Build history of the part. All positions in model axes, mm. Face numbers are marked on the shaded views. Round coordinates to 2 decimals unless told otherwise and drop trailing zeros. Loops run counter-clockwise (first coordinate to the right, second up) from the corner with the lowest first, then second, coordinate; pieces in that order, holes last. Notation, with made-up numbers: (20.25, 81.25) - (50.25, 81.25) arc R24 cw to (50.25, 91.25) - close; hole circle Ø5 at (43, 89.5). An arc over 180 degrees is marked (long way). Use one line per item in the form item = value. Start each with the question number.
Q1. Saw through at A-A (z = 0). Give the cut face in (x, y).
Q2. Saw through at B-B (x = 0). Give the cut face in (y, z).
Q3. Drill centre lines: line 1 (Y direction, x = -22, z = -29.5); line 2 (Z direction, x = 10.5, y = 2.75); line 3 (X direction, y = 2.5, z = 14). Where is each one in solid material? Low to high.
Q4. Mould opens along X. For the marked faces 1, 2 and 3 say: released by +X, released by -X, zero draft, split by the parting line, or undercut.
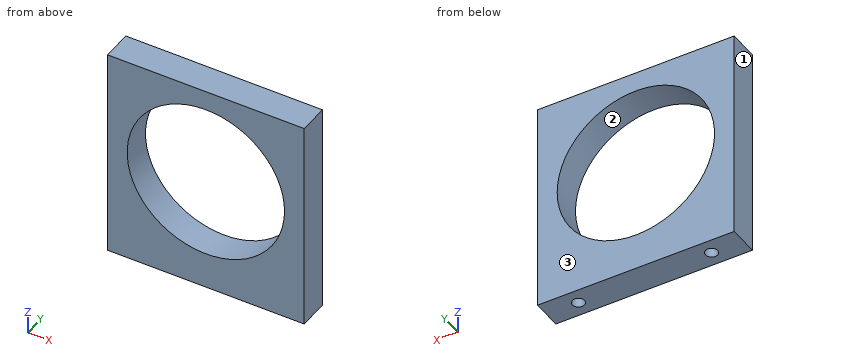
```python
from build123d import *

# Parameters (mm, degrees)
F0_W     = 65
F0_H     = 70.5
F0_R     = 26
F1_DEPTH = 5
F3_D     = 4
F3_DEPTH = 15
F3_TIP   = 1.2017212381


with BuildPart() as f1:
    # F0 (on Front) → F1 (new body, symmetric)
    with BuildSketch(Plane.XZ):
        with Locations((0, -2.75)):
            Rectangle(F0_W, F0_H)
        Circle(F0_R, mode=Mode.SUBTRACT)
    extrude(amount=F1_DEPTH, both=True)

    # F3
    with Locations(Plane(origin=(0, 0, -38), x_dir=(1, 0, 0), z_dir=(0, 0, -1))):
        with Locations((-22, 0), (22, 0)):
            Hole(F3_D / 2, depth=F3_DEPTH)
            with Locations((0, 0, -(F3_DEPTH + F3_TIP / 2))):  # 118° drill point
                Cone(0, F3_D / 2, F3_TIP, mode=Mode.SUBTRACT)


solid = f1.part
```
Report:
q1.outline = (-32.5, -5) - (-26, -5) - (-26, 5) - (-32.5, 5) - close; (26, -5) - (32.5, -5) - (32.5, 5) - (26, 5) - close
q2.outline = (-5, -38) - (5, -38) - (5, -26) - (-5, -26) - close; (-5, 26) - (5, 26) - (5, 32.5) - (-5, 32.5) - close
q3.line_1 = -5 to -2, 2 to 5
q3.line_2 = -38 to -23.79, 23.79 to 32.5
q3.line_3 = -32.5 to -21.91, 21.91 to 32.5
q4.face_1 = released by -X
q4.face_2 = undercut
q4.face_3 = zero draft
